Read the model definition and answer for the solid it produces. Units are mm, in the model's axes. Round coordinates to 2 decimals unless told otherwise and drop trailing zeros. Order: outer loops, then holes, each group sorted by start corner. A loop starts at its lowest first (then second) coordinate and runs counter-clockwise, first axis right, second up. Notation, with made-up numbers: M 29,35 L 54,35 A26 ccw 54,51 Z; hole C 48,39 d11. An arc over 180 degrees is marked long. Answer as CSV lines item,"result".
```python
from build123d import *

# Parameters (mm, degrees)
F0_R     = 22.225
F1_DEPTH = 25.4
F2_SIZE  = 2.54


with BuildPart() as f1:
    # F0 (on Front) → F1 (new body)
    with BuildSketch(Plane.XZ):
        Polygon((-36.271735, 16.149217), (-39.704357, 0), (-36.271735, -16.149217), (-26.5674, -29.506087), (-12.269321, -37.761087), (4.150235, -39.486852), (19.852179, -34.384982), (32.1215, -23.337636), (38.836722, -8.255), (38.836722, 8.255), (32.1215, 23.337636), (19.852179, 34.384982), (4.150235, 39.486852), (-12.269321, 37.761087), (-26.5674, 29.506087), align=None)
        Circle(F0_R, mode=Mode.SUBTRACT)
    extrude(amount=F1_DEPTH)

    # F2
    f2_edges = [f1.edges().sort_by_distance(p)[0] for p in [
        (35.479111, -25.4, -15.796318),
        (38.836722, -25.4, 0),
        (35.479111, -25.4, 15.796318),
        (25.986839, -25.4, 28.861309),
        (12.001207, -25.4, 36.935917),
        (-4.059543, -25.4, 38.62397),
        (-19.418361, -25.4, 33.633587),
        (-31.419568, -25.4, 22.827652),
        (-37.988046, -25.4, 8.074608),
        (-37.988046, -25.4, -8.074608),
        (-31.419568, -25.4, -22.827652),
        (-19.418361, -25.4, -33.633587),
        (-4.059543, -25.4, -38.62397),
        (12.001207, -25.4, -36.935917),
        (25.986839, -25.4, -28.861309),
        (-22.225, -25.4, 0),
        (35.479111, 0, -15.796318),
        (38.836722, 0, 0),
        (35.479111, 0, 15.796318),
        (25.986839, 0, 28.861309),
        (12.001207, 0, 36.935917),
        (-4.059543, 0, 38.62397),
        (-19.418361, 0, 33.633587),
        (-31.419568, 0, 22.827652),
        (-37.988046, 0, 8.074608),
        (-37.988046, 0, -8.074608),
        (-31.419568, 0, -22.827652),
        (-19.418361, 0, -33.633587),
        (-4.059543, 0, -38.62397),
        (12.001207, 0, -36.935917),
        (25.986839, 0, -28.861309),
        (-22.225, 0, 0),
    ]]
    chamfer(f2_edges, length=F2_SIZE)


solid = f1.part
```
Item 1: Flat-ended cylindrical pins translate along their axes: pin 1 (6 mm diameter, centred on x = 22.5, y = -12, fed in from +Z); pin 2 (10 mm diameter, centred on y = -12.5, z = -17, fed in from -X); pin 3 (4 mm diameter, centred on y = -22, z = -10, fed in from -X). Find the tip coordinate at first contact, or state that the pin passes through.
Ans:
pin 1,"z = 34.5"
pin 2,"x = -37.15"
pin 3,"x = -38"
Item 2: Find the intervals of material crossed by probe 1 along Z at (x, y) = (0, -7.75) (3 decimals); probe 2 along X at (y, z) = (-18.5, -7); probe 3 along X at (y, z) = (-3.75, 6.5), in increasing order. Write a range as [from, to].
Ans:
probe 1,"[-39.051, -22.225], [22.225, 39.051]"
probe 2,"[-38.22, -21.09], [21.09, 38.84]"
probe 3,"[-38.32, -21.25], [21.25, 38.84]"
Item 3: A cutting plane is placed at C-C, the plane x = 27.5. Determine the outline of the cut face in (y, z).
Ans:
outline,"M -25.4,-24.08 L -22.86,-27.5 L -2.54,-27.5 L 0,-24.08 L 0,24.08 L -2.54,27.5 L -22.86,27.5 L -25.4,24.08 Z"
Item 4: A cutting plane is placed at B-B, the plane x = 0. Determine the outline of the cut face in (y, z) (3 decimals).
Ans:
outline,"M -25.4,-36.497 L -22.86,-39.051 L -2.54,-39.051 L 0,-36.497 L 0,-24.765 L -2.54,-22.225 L -22.86,-22.225 L -25.4,-24.765 Z; M -25.4,24.765 L -22.86,22.225 L -2.54,22.225 L 0,24.765 L 0,36.497 L -2.54,39.051 L -22.86,39.051 L -25.4,36.497 Z"
Item 5: Determine the mould class of faces 1 (the face through (25.04, -1.25, -27.98)), 2 (the face through (21.35, -2.38, 6.72)), 3 (the face through (11.713, -1.252, 35.675)) for opening direction Z: +Z half, -Z half, draft (parallel to the pull), parting line (faces both ways), or undercut.
Ans:
face 1,"-Z half"
face 2,"undercut"
face 3,"+Z half"
